from build123d import *

# Parameters (mm, degrees)
BOSS_EXTRUDE1_DEPTH = 6.35
SKETCH2_R           = 2.4
SKETCH2_R_2         = 4.9
CUT_EXTRUDE1_DEPTH  = 170.824387236
SKETCH5_R           = 1.05
CUT_EXTRUDE2_DEPTH  = 170.824387236


with BuildPart() as part:
    # Sketch1 → Boss-Extrude1 (new body)
    with BuildSketch(Plane(origin=(0, 0, 0), x_dir=(1, 0, 0), z_dir=(0, 1, 0))):
        with BuildLine():
            Line((10, 0), (110, 0))
            ThreePointArc((110, 0), (117.071067812, 2.928932188), (120, 10))
            Line((120, 10), (120, 110))
            ThreePointArc((120, 110), (117.071067812, 117.071067812), (110, 120))
            Line((110, 120), (10, 120))
            ThreePointArc((10, 120), (2.928932188, 117.071067812), (0, 110))
            Line((0, 110), (0, 10))
            ThreePointArc((0, 10), (2.928932188, 2.928932188), (10, 0))
        make_face()
    extrude(amount=BOSS_EXTRUDE1_DEPTH)

    # Sketch2 → Cut-Extrude1 (cut, through all)
    with BuildSketch(Plane(origin=(0, 6.35, 0), x_dir=(1, 0, 0), z_dir=(0, 1, 0))):
        with Locations(Location((59.326447526, 12.4, 0), (0, 0, 270))):
            Circle(SKETCH2_R)
        with Locations(Location((96.90831454, 12.4, 0), (0, 0, 270))):
            Circle(SKETCH2_R)
        with Locations(Location((106.276743553, 88.69973137, 0), (0, 0, 270))):
            Circle(SKETCH2_R)
        with Locations(Location((10, 110, 0), (0, 0, 270))):
            Circle(SKETCH2_R_2)
        with Locations(Location((10, 10, 0), (0, 0, 270))):
            Circle(SKETCH2_R_2)
        with Locations(Location((110, 110, 0), (0, 0, 270))):
            Circle(SKETCH2_R_2)
        with Locations(Location((110, 10, 0), (0, 0, 270))):
            Circle(SKETCH2_R_2)
        Polygon((57.291464341, 23.213164461), (74.324967949, 12.731764037), (112.886040109, 75.398023809), (95.852536501, 85.879424234), align=None)
    extrude(amount=-CUT_EXTRUDE1_DEPTH, mode=Mode.SUBTRACT)

    # Sketch5 → Cut-Extrude2 (cut, through all)
    with BuildSketch(Plane(origin=(0, 6.35, 0), x_dir=(1, 0, 0), z_dir=(0, 1, 0))):
        with Locations(Location((66.679748999, 51.827220643, 0), (0, 0, 270))):
            Circle(SKETCH5_R)
        with Locations(Location((56.459646835, 58.116060898, 0), (0, 0, 270))):
            Circle(SKETCH5_R)
        with Locations(Location((74.540799318, 64.602348349, 0), (0, 0, 270))):
            Circle(SKETCH5_R)
        with Locations(Location((64.320697153, 70.891188603, 0), (0, 0, 270))):
            Circle(SKETCH5_R)
        with Locations(Location((10.796792254, 85.040096841, 0), (0, 0, 270))):
            Circle(SKETCH5_R)
        with Locations(Location((21.016894418, 78.751256587, 0), (0, 0, 270))):
            Circle(SKETCH5_R)
        with Locations(Location((29.926084779, 93.229734653, 0), (0, 0, 270))):
            Circle(SKETCH5_R)
        with Locations(Location((19.705982614, 99.518574908, 0), (0, 0, 270))):
            Circle(SKETCH5_R)
    extrude(amount=-CUT_EXTRUDE2_DEPTH, mode=Mode.SUBTRACT)


solid = part.part
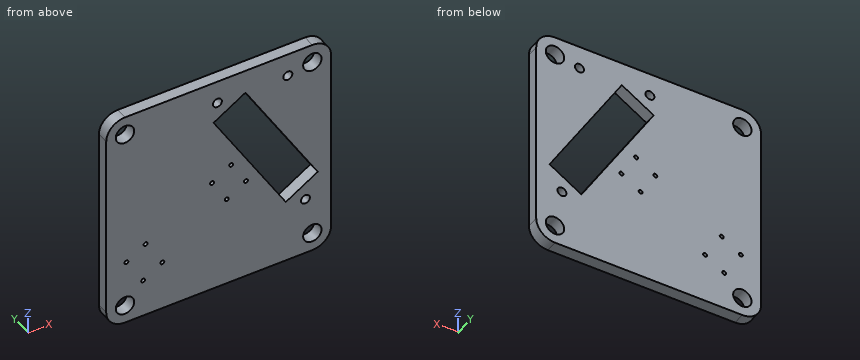
CAD build for the part. Positions are in the model's coordinates, mm. Coordinates: 2 decimals unless noted, no trailing zeros. Loops run counter-clockwise (first coordinate to the right, second up) from the corner with the lowest first, then second, coordinate; pieces in that order, holes last. Notation, with made-up numbers: (65.5, 41.25) - (95.5, 41.25) arc R24 ccw to (95.5, 60.25) - close; hole circle Ø11 at (28, 50.25). An arc over 180 degrees is marked (long way). Use one line per item in the form item = value. Start each with the question number.
1) Band-saw the part on A-A (z = -29.5). Give the cut face in (x, y), and give its area (3 significant figures).
2) Flat gauge pin, fed straight in: pin 1 (1.7 mm diameter, centred on x = 10.8, z = -85.04, fed in from -Y). Where does the tip first touch, or does it go through?
3) Band-saw the part on D-D (z = -108). Give the cut face in (x, y).
4) Band-saw the part on B-B (x = 80). Give the cut face in (y, z), and give its area (3 significant figures).
5) Drill centre lines: L1, parallel to X at y = 5.75, z = -110.5; L2, parallel to Z at x = 112, y = 0.75; L3, parallel to Z at x = 114.5, y = 0.5. Where is each one in solid material? Low to high. Write a range as from..to.
6) Band-saw the part on C-C (y = 2). State how many separate pieces and enclosed holes the cut face has, and give its area (3 significant figures).
Check values:
q1.outline = (0, 0) - (61.16, 0) - (61.16, 6.35) - (0, 6.35) - close; (84.64, 0) - (120, 0) - (120, 6.35) - (84.64, 6.35) - close
q1.area = 613 mm2
q2.pin_1 = through
q3.outline = (0, 0) - (5.53, 0) - (5.53, 6.35) - (0, 6.35) - close; (14.47, 0) - (105.53, 0) - (105.53, 6.35) - (14.47, 6.35) - close; (114.47, 0) - (120, 0) - (120, 6.35) - (114.47, 6.35) - close
q4.outline = (0, -120) - (6.35, -120) - (6.35, -60.12) - (0, -60.12) - close; (0, -21.95) - (6.35, -21.95) - (6.35, 0) - (0, 0) - close
q4.area = 520 mm2
q5.L1 = 0.01..5.13, 14.87..105.13, 114.87..119.99
q5.L2 = -119.8..-114.47, -105.53..-75.94, -73.96..-14.47, -5.53..-0.2
q5.L3 = -118.93..-111.94, -108.06..-11.94, -8.06..-1.07
q6.separate_pieces = 1
q6.enclosed_holes = 16
q6.area = 12,500 mm2
